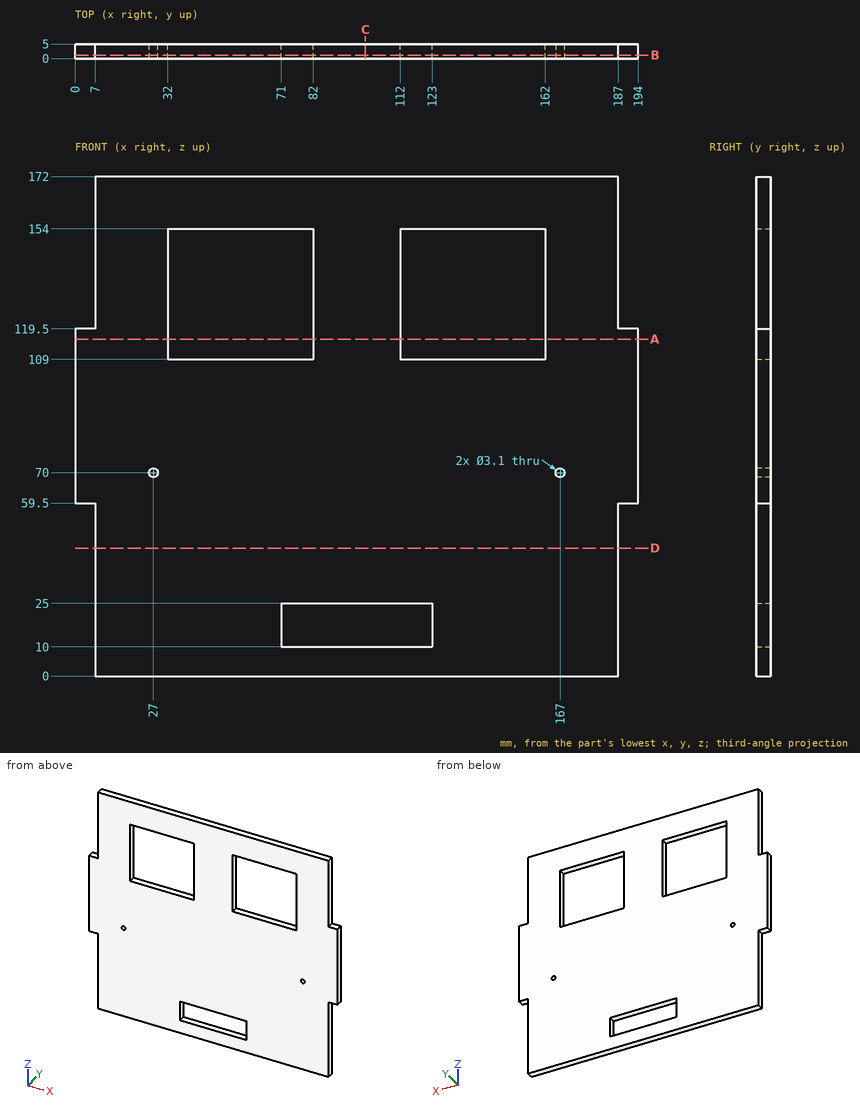
Could you check a few things on this drawing? It's one solid part, dimensions in mm from its lowest x, y, z. Round coordinates to 2 decimals unless told otherwise and drop trailing zeros. Order: outer loops, then holes, each group sorted by start corner. A loop starts at its lowest first (then second) coordinate and runs counter-clockwise, first axis right, second up. Notation, with made-up numbers: M -20.75,43 L 20.25,43 A24 ccw 20.25,70 Z; hole C -31.75,9.25 d9. An arc over 180 degrees is marked long. One line per item, written item: value.
(1) I need wall thicknesses on line 1 along X through (y, z) = (3.7, 138); line 2 along Z through (x, y) = (77, 1.6); line 3 along X through (y, z) = (3, 70). Which ranges of each line are inside material? Lowest first, please. Write a range as from..to.
Ans:
line 1: x = 7..32, 82..112, 162..187
line 2: z = 0..10, 25..109, 154..172
line 3: x = 0..25.45, 28.55..165.45, 168.55..194
(2) Imagine slicing it at C-C (x = 100). Write out the boundary of the cut face in (y, z).
Ans:
outline: M 0,0 L 5,0 L 5,10 L 0,10 Z; M 0,25 L 5,25 L 5,172 L 0,172 Z
(3) I'm going to push flat-ended pins straight in: P1, Ø2.5, axis at y = 3.5, z = 134, coming from the +X side; P2, Ø2.5, axis at x = 191, y = 2.5, coming from the +Z side; P3, Ø2.5, axis at y = 2, z = 18, coming from the -X side. Where does each tip first touch, or does it pass through?
Ans:
P1: stops at x = 187
P2: stops at z = 119.5
P3: stops at x = 7
(4) Imagine slicing it at A-A (z = 116). Write out the boundary of the cut face in (x, y).
Ans:
outline: M 0,0 L 32,0 L 32,5 L 0,5 Z; M 82,0 L 112,0 L 112,5 L 82,5 Z; M 162,0 L 194,0 L 194,5 L 162,5 Z
(5) Imagine slicing it at B-B (y = 1.15). Write out the boundary of the cut face in (x, z), and give its area (3 significant figures).
Ans:
outline: M 0,59.5 L 7,59.5 L 7,0 L 187,0 L 187,59.5 L 194,59.5 L 194,119.5 L 187,119.5 L 187,172 L 7,172 L 7,119.5 L 0,119.5 Z; hole C 27,70 d3.1; hole M 32,109 L 82,109 L 82,154 L 32,154 Z; hole M 71,10 L 123,10 L 123,25 L 71,25 Z; hole M 112,109 L 162,109 L 162,154 L 112,154 Z; hole C 167,70 d3.1
area: 26,500 mm^2
(6) Imagine slicing it at D-D (z = 44). Write out the boundary of the cut face in (x, y), and give its area (3 significant figures).
Ans:
outline: M 7,0 L 187,0 L 187,5 L 7,5 Z
area: 900 mm^2
